Could you check a few things on this model? Use its own coordinates, in mm. A direction names the side the tool comes from. Give positions to 0.01 mm unless a question says otherwise; leave off trailing zeros. Loops run counter-clockwise (first coordinate to the right, second up) from the corner with the lowest first, then second, coordinate; pieces in that order, holes last. Notation, with made-up numbers: M 83,2.5 L 92,2.5 A27 ccw 92,25.5 Z; hole C 82,-13.75 d9. An arc over 180 degrees is marked long. Return JSON: item names as keys, results as strings. Group by question number.
1. Please list where these lines run through material, in increasing order: line 1 (Y direction, x = -12.66, z = 0.6); line 2 (X direction, y = 34.5, z = 1.7); line 3 (X direction, y = -34, z = 1.9).
2. If we section it at C-C (x = -36.5): Write out the boundary of the cut face in (y, z).
3. If we mould it in two halves opening along Y, with no side actions, what happens to faces 4 (the cylindrical face through (-1.1, 39.94, 1.48)), 5 (the cylindrical face through (-96.81, 0.11, 1.48)), 6 (the flat face through (-36.975, -27.298, 1.479))? For each: +Y half, -Y half, draft (parallel to the pull), parting line (faces both ways), or undercut.
4. If we section it at B-B (y = -14.5): Write out the boundary of the cut face in (x, z), plus the area to 3 significant figures.
5. If we section it at A-A (z = 0.45): State how many separate pieces and enclosed holes the cut face has, plus the area to 3 significant figures.
6. For faces 1 (the cylindrical face through (-1.4, -14.9, 1.5)), 2 (the cylindrical face through (-106.02, 2.41, 1.48)), 3 (the flat face through (-79, -10.003, 1)), which set-ups out of +Z, -Z, +X, -X, +Y, -Y let a thin tool reach every point of the face, with its end or its side?
7. For pin 1 (1 mm diameter, centred on y = 18, z = 1.5, fed in from +X); pin 2 (1.5 mm diameter, centred on x = -71, z = 2, fed in from -Y); pin 3 (0.9 mm diameter, centred on y = 3, z = 1, fed in from +X), each with a flat end and sliding along its axis, tell me the tip position at first contact or that it passes through.
```python
from build123d import *

# Parameters (mm, degrees)
SKETCH1_R           = 2.55
BOSS_EXTRUDE2_DEPTH = 3


with BuildPart() as part:
    # Sketch1 → Boss-Extrude2 (new body)
    with BuildSketch(Plane.XY):
        with BuildLine():
            Line((0, 20.000781807), (0, 35.380781807))
            ThreePointArc((0, 35.380781807), (-1.131516477, 40.001387827), (-4.27, 43.576335479))
            ThreePointArc((-4.27, 43.576335479), (-11.306226361, 46.201792614), (-18.733195752, 45.087507084))
            Line((-18.733195752, 45.087507084), (-98.964962039, 10.981553375))
            ThreePointArc((-98.964962039, 10.981553375), (-106.051053982, 2.24930594), (-102.807556787, -8.518450105))
            ThreePointArc((-102.807556787, -8.518450105), (-101.178529417, -9.616994075), (-99.252006076, -10.003046978))
            Line((-99.252006076, -10.003046978), (-58.412006076, -10.003046978))
            ThreePointArc((-58.412006076, -10.003046978), (-54.585171753, -10.764251653), (-51.340938265, -12.931979166))
            Line((-51.340938265, -12.931979166), (-22.201067812, -42.071849618))
            ThreePointArc((-22.201067812, -42.071849618), (-18.956834324, -44.239577132), (-15.13, -45.000781807))
            Line((-15.13, -45.000781807), (-10, -45.000781807))
            ThreePointArc((-10, -45.000781807), (-2.928932188, -42.071849618), (0, -35.000781807))
            Line((0, -35.000781807), (0, -20.000781807))
            ThreePointArc((0, -20.000781807), (-1.468196752, -14.784621022), (-5.441666667, -11.100130301))
            ThreePointArc((-5.441666667, -11.100130301), (-6.23636065, -10.363232157), (-6.53, -9.32))
            Line((-6.53, -9.32), (-6.53, 9.32))
            ThreePointArc((-6.53, 9.32), (-6.23636065, 10.363232157), (-5.441666667, 11.100130301))
            ThreePointArc((-5.441666667, 11.100130301), (-1.468196752, 14.784621022), (0, 20.000781807))
        make_face()
        with Locations((-94.264328129, -0.003046978)):
            Circle(SKETCH1_R, mode=Mode.SUBTRACT)
        with Locations((-72.164328129, -0.003046978)):
            Circle(SKETCH1_R, mode=Mode.SUBTRACT)
        with Locations((-14.564328129, -0.003046978)):
            Circle(SKETCH1_R, mode=Mode.SUBTRACT)
        with Locations((-12.66, 35.499218193)):
            Circle(SKETCH1_R, mode=Mode.SUBTRACT)
        with Locations((-12.66, -35.500781807)):
            Circle(SKETCH1_R, mode=Mode.SUBTRACT)
    extrude(amount=BOSS_EXTRUDE2_DEPTH)


solid = part.part
```
Answer:
{
 "1": {"line 1": "y = -45 to -38.05, -32.95 to -1.7, 1.69 to 32.95, 38.05 to 46.28", "line 2": "x = -43.64 to -15.01, -10.31 to 0", "line 3": "x = -30.27 to -14.72, -10.6 to 0"},
 "2": {"outline": "M -27.77,0 L 37.53,0 L 37.53,3 L -27.77,3 Z"},
 "3": {"face 4": "+Y half", "face 5": "undercut", "face 6": "-Y half"},
 "4": {"outline": "M -49.77,0 L -1.65,0 L -1.65,3 L -49.77,3 Z", "area": "144 mm²"},
 "5": {"separate pieces": "1", "enclosed holes": "5", "area": "5,180 mm²"},
 "6": {"face 1": "+Z, -Z, +X", "face 2": "+Z, -Z, -X", "face 3": "+Z, -Z, -X, -Y"},
 "7": {"pin 1": "stops at x = -0.11", "pin 2": "stops at y = -10", "pin 3": "stops at x = -6.53"}
}
